```python
from build123d import *

# Parameters (mm, degrees)
BOSS_EXTRUDE1_DEPTH = 32.5
CHAMFER1_SIZE       = 5
SKETCH2_R           = 5
CUT_EXTRUDE1_DEPTH  = 10
SKETCH3_R           = 5
BOSS_EXTRUDE2_DEPTH = 10


with BuildPart() as part:
    # Sketch1 → Boss-Extrude1 (new body, symmetric)
    with BuildSketch(Plane.XY):
        with BuildLine():
            Line((47.428571429, 0), (47.428571429, -40))
            Line((47.428571429, -40), (-32.571428571, -40))
            ThreePointArc((-32.571428571, -40), (-52.571428571, -20), (-32.571428571, 0))
            Line((-32.571428571, 0), (-26.571428571, 0))
            ThreePointArc((-26.571428571, 0), (-8.071428571, 12.400657923), (10.428571429, 0))
            Line((10.428571429, 0), (47.428571429, 0))
        make_face()
    extrude(amount=BOSS_EXTRUDE1_DEPTH, both=True)

    # Chamfer1
    chamfer1_edges = [part.edges().sort_by_distance(p)[0] for p in [
        (28.928571429, 0, 32.5),
        (-8.071428571, 12.400657923, 32.5),
        (-29.571428571, 0, 32.5),
        (-52.571428571, -20, 32.5),
        (-29.571428571, 0, -32.5),
        (-8.071428571, 12.400657923, -32.5),
        (28.928571429, 0, -32.5),
        (7.428571429, -40, -32.5),
        (-52.571428571, -20, -32.5),
        (7.428571429, -40, 32.5),
    ]]
    chamfer(chamfer1_edges, length=CHAMFER1_SIZE)

    # Sketch2 → Cut-Extrude1 (cut)
    with BuildSketch(Plane.XY.offset(32.5)):
        with Locations((-8.071428571, -20)):
            Circle(SKETCH2_R)
    extrude(amount=-CUT_EXTRUDE1_DEPTH, mode=Mode.SUBTRACT)

    # Sketch3 → Boss-Extrude2 (add)
    with BuildSketch(Plane(origin=(47.428571429, 0, 0), x_dir=(0, 0, -1), z_dir=(1, 0, 0))):
        with Locations((0, -20)):
            Circle(SKETCH3_R)
    extrude(amount=BOSS_EXTRUDE2_DEPTH)


solid = part.part
```
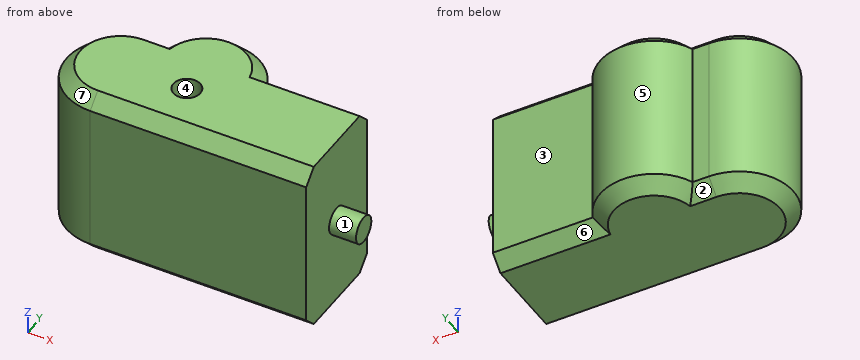
Source: CAD feature listing. Evaluate the final solid. Frame: model axes, mm. Face numbers are marked on the shaded views. A direction names the side the tool comes from. Round coordinates to 2 decimals unless told otherwise and drop trailing zeros. Order: outer loops, then holes, each group sorted by start corner. A loop starts at its lowest first (then second) coordinate and runs counter-clockwise, first axis right, second up. Notation, with made-up numbers: (7, 54) -> (33, 54) arc R14 ccw to (33, 72) -> close; hole circle Ø3 at (15.5, 13). An arc over 180 degrees is marked (long way). One line per item, written item: value. Start each with the question number.
Q1. Material intervals for probe 1 along Y at (x, z) = (19, -25.5); probe 2 along X at (y, z) = (-4, -11); probe 3 along X at (y, z) = (-38, 22.5), sorted ascending.
Q2. Section query B-B (x = 36.5). Return the cut outline in (y, z), plus the area to 3 significant figures.
Q3. Section query C-C (y = -20). Return the cut outline in (x, z), plus the area to 4 significant figures.
Q4. Pin query (flat end, axial travel): pin 1 (1.8 mm diameter, centred on x = -30, z = -3, fed in from +Y); pin 2 (10 mm diameter, centred on y = -1, z = 10.5, fed in from +X); pin 3 (8 mm diameter, centred on y = -30.5, z = 4, fed in from -X); pin 4 (1.5 mm diameter, centred on x = -40.5, y = -7, fed in from +Z). Return the tip coordinate at first contact, or that it passes through.
Q5. Draft query along X for the marked faces 4, 5, 6 and 7. Return one class per face: pulls with the +X half, pulls with the -X half, needs draft (parallel to the pull), parting line crosses it, or undercut.
Q6. Section query D-D (z = 16.5). Return the cut outline in (x, y), plus the area to 3 significant figures.
Q7. Section query A-A (z = 0). Return the cut outline in (x, y).
Q8. Access query for the marked faces 1, 2 and 3. Directions: +Z, -Z, +X, -X, +Y, -Y. A direction counts if a zero-diameter tool reaches every point of the face in a straight line with its end or side. Return the directions, or none.
Findings below:
1. probe 1: -40 to 0
1. probe 2: -44.57 to 47.43
1. probe 3: -41.29 to 47.43
2. outline: (-40, -27.5) -> (-35, -32.5) -> (-5, -32.5) -> (0, -27.5) -> (0, 27.5) -> (-5, 32.5) -> (-35, 32.5) -> (-40, 27.5) -> close
2. area: 2,550 mm²
3. outline: (-52.57, -27.5) -> (-47.57, -32.5) -> (47.43, -32.5) -> (47.43, -5) -> (57.43, -5) -> (57.43, 5) -> (47.43, 5) -> (47.43, 32.5) -> (-3.07, 32.5) -> (-3.07, 22.5) -> (-13.07, 22.5) -> (-13.07, 32.5) -> (-47.57, 32.5) -> (-52.57, 27.5) -> close
3. area: 6,475 mm²
4. pin 1: y = 0
4. pin 2: x = 47.43
4. pin 3: x = -51.49
4. pin 4: z = 32.5
5. face 4: undercut
5. face 5: parting line crosses it
5. face 6: needs draft
5. face 7: pulls with the -X half
6. outline: (-32.57, -40) -> (47.43, -40) -> (47.43, 0) -> (10.43, 0) arc R20 ccw to (-26.57, 0) -> (-32.57, 0) arc R20 ccw to start
6. area: 4,160 mm²
7. outline: (-32.57, -40) -> (47.43, -40) -> (47.43, -25) -> (57.43, -25) -> (57.43, -15) -> (47.43, -15) -> (47.43, 0) -> (10.43, 0) arc R20 ccw to (-26.57, 0) -> (-32.57, 0) arc R20 ccw to start
8. face 1: +X
8. face 2: -Z, -X, +Y
8. face 3: +Z, -Z, +X, +Y
